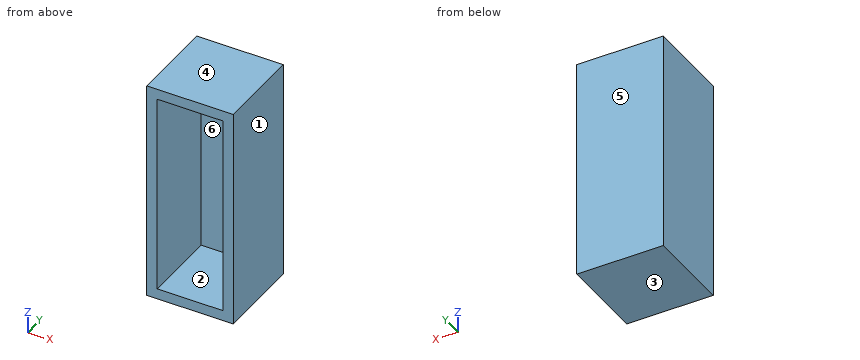
from build123d import *

# Parameters (mm, degrees)
F0_W     = 419.1
F0_H     = 419.1
F1_DEPTH = 1073.15
F2_T     = -50.8
F3_W     = 317.5
F3_H     = 152.4
F4_DEPTH = 19.05


with BuildPart() as f1:
    # F0 (on Top) → F1 (new body)
    with BuildSketch(Plane.XY):
        with Locations((0.943545, 59.428082)):
            Rectangle(F0_W, F0_H)
    extrude(amount=F1_DEPTH)

    # F2
    f2_openings = [f1.faces().sort_by_distance(p)[0] for p in [
        (0.943545, -150.121918, 536.575),
    ]]
    offset(amount=F2_T, openings=f2_openings)

    # F3 (on face) → F4 (join)
    with BuildSketch(Plane.XZ.offset(-218.178082)):
        with Locations((0.943545, 946.15)):
            Rectangle(F3_W, F3_H)
    extrude(amount=F4_DEPTH)


solid = f1.part
Part model, mm, in its own coordinate system. Face numbers are marked on the shaded views. A direction names the side the tool comes from. Give positions to 0.01 mm unless a question says otherwise; leave off trailing zeros. Write each loop counter-clockwise with the first axis right and the second up, starting at its lowest first coordinate (ties: lowest second). Pieces come first, ordered by that corner, then holes.
1) Probe L1, parallel to X at y = -96, z = 534; L2, parallel to Z at x = -146.5, y = -2.5; L3, parallel to Y at x = -146, z = 893.5. List the from-to ranges inside material, lowest first.
Resolved:
L1: x = -208.61 to -157.81, 159.69 to 210.49
L2: z = 0 to 50.8, 1022.35 to 1073.15
L3: y = 199.13 to 268.98
2) Cut at A-A on y = -68. Write the cut outline in (x, z).
Resolved:
outline: (-208.61, 0) - (210.49, 0) - (210.49, 1073.15) - (-208.61, 1073.15) - close; hole (-157.81, 50.8) - (159.69, 50.8) - (159.69, 1022.35) - (-157.81, 1022.35) - close
3) Cut at B-B on z = 847. Write the cut outline in (x, y).
Resolved:
outline: (-208.61, -150.12) - (-157.81, -150.12) - (-157.81, 218.18) - (159.69, 218.18) - (159.69, -150.12) - (210.49, -150.12) - (210.49, 268.98) - (-208.61, 268.98) - close
4) Which spindle directions (+Z, -Z, +X, -X, +Y, -Y) get a long thin tool onto all of the face, cutting with end or side? Do the marked faces 1 and 2. Say none if no direction does.
Resolved:
face 1: +Z, -Z, +X, +Y, -Y
face 2: -Y
5) Two-plate mould, pull along Z, no slides. Class the marked faces 3, 4, 5 and 6: released by +Z, released by -Z, zero draft, split by the parting line, or undercut.
Resolved:
face 3: released by -Z
face 4: released by +Z
face 5: zero draft
face 6: undercut
6) Cut at C-C on x = 127. Write the cut outline in (y, z), then the cut area to 3 significant figures.
Resolved:
outline: (-150.12, 0) - (268.98, 0) - (268.98, 1073.15) - (-150.12, 1073.15) - (-150.12, 1022.35) - (199.13, 1022.35) - (199.13, 869.95) - (218.18, 869.95) - (218.18, 50.8) - (-150.12, 50.8) - close
area: 94,800 mm2
